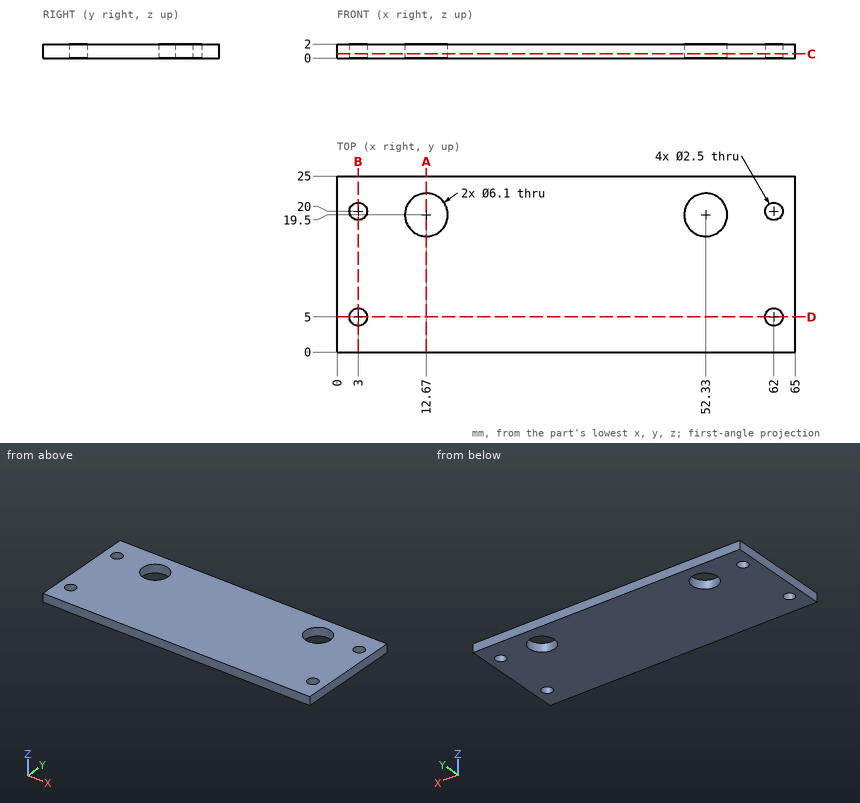
Verification items for this drawing (mm, ordinates from the low corner). Coordinates: 2 decimals unless noted, no trailing zeros. Write each loop counter-clockwise with the first axis right and the second up, starting at its lowest first coordinate (ties: lowest second). Pieces come first, ordered by that corner, then holes. Notation, with made-up numbers: M 32.5,13 L 72.5,13 A22 ccw 72.5,33 Z; hole C 83,89.5 d4. An arc over 180 degrees is marked long. Answer as a JSON object with one key per item and string values. Group by question number.
(1) Cross-section at A-A, the plane x = 12.67. Record the cut outline in (y, z), and give its area (3 significant figures).
(2) Cross-section at B-B, the plane x = 3. Record the cut outline in (y, z), and give its area (3 significant figures).
(3) Cross-section at D-D, the plane y = 5. Record the cut outline in (x, z).
(4) Cross-section at C-C, the plane z = 0.6. Record the cut outline in (x, y).
(5) Gauge pin test, flat end, axial feed: pin 1 (3 mm diameter, centred on x = 3, y = 5, fed in from +Z). Record the tip position at first contact, or that the pin passes through.
(6) Material ranges on line 1 (Y direction, x = 62, z = 0.8); line 2 (Y direction, x = 52.33, z = 1.35); line 3 (X direction, y = 4.5, z = 1.05), recorded low to high.
Reply:
{
 "1": {"outline": "M 0,0 L 16.45,0 L 16.45,2 L 0,2 Z; M 22.55,0 L 25,0 L 25,2 L 22.55,2 Z", "area": "37.8 mm²"},
 "2": {"outline": "M 0,0 L 3.75,0 L 3.75,2 L 0,2 Z; M 6.25,0 L 18.75,0 L 18.75,2 L 6.25,2 Z; M 21.25,0 L 25,0 L 25,2 L 21.25,2 Z", "area": "40.0 mm²"},
 "3": {"outline": "M 0,0 L 1.75,0 L 1.75,2 L 0,2 Z; M 4.25,0 L 60.75,0 L 60.75,2 L 4.25,2 Z; M 63.25,0 L 65,0 L 65,2 L 63.25,2 Z"},
 "4": {"outline": "M 0,0 L 65,0 L 65,25 L 0,25 Z; hole C 3,5 d2.5; hole C 3,20 d2.5; hole C 12.67,19.5 d6.1; hole C 52.33,19.5 d6.1; hole C 62,5 d2.5; hole C 62,20 d2.5"},
 "5": {"pin 1": "z = 2"},
 "6": {"line 1": "0 to 3.75, 6.25 to 18.75, 21.25 to 25", "line 2": "0 to 16.45, 22.55 to 25", "line 3": "0 to 1.85, 4.15 to 60.85, 63.15 to 65"}
}
